```python
from build123d import *

# Parameters (mm, degrees)
SKETCH1_W           = 28.4
SKETCH1_H           = 40.1
BOSS_EXTRUDE1_DEPTH = 4.75
SKETCH2_W           = 3.4
SKETCH2_H           = 23.1
SKETCH2_H_2         = 30.1
CUT_EXTRUDE1_DEPTH  = 26.024088395
SKETCH4_W           = 13.85
SKETCH4_H           = 38.1
SKETCH4_W_2         = 7.85
SKETCH4_H_2         = 30.1
BOSS_EXTRUDE2_DEPTH = 4


with BuildPart() as part:
    # Sketch1 → Boss-Extrude1 (new body)
    with BuildSketch(Plane.XY):
        Rectangle(SKETCH1_W, SKETCH1_H)
    extrude(amount=BOSS_EXTRUDE1_DEPTH)

    # Sketch2 → Cut-Extrude1 (cut, through all)
    with BuildSketch(Plane.XY.offset(4.75)):
        with Locations((10.5, 0)):
            Rectangle(SKETCH2_W, SKETCH2_H)
        with Locations((-10.5, 0)):
            Rectangle(SKETCH2_W, SKETCH2_H)
        Rectangle(SKETCH2_W, SKETCH2_H_2)
    extrude(amount=-CUT_EXTRUDE1_DEPTH, mode=Mode.SUBTRACT)

    # Sketch4 → Boss-Extrude2 (add)
    with BuildSketch(Plane(origin=(0, 0, 0), x_dir=(-1, 0, 0), z_dir=(0, 0, -1))):
        with Locations((0, 1)):
            Rectangle(SKETCH4_W, SKETCH4_H)
        Rectangle(SKETCH4_W_2, SKETCH4_H_2, mode=Mode.SUBTRACT)
    extrude(amount=BOSS_EXTRUDE2_DEPTH)


solid = part.part
```
Can you work these out from the model? Positions are in its coordinate system, mm. A direction names the side the tool comes from. Round coordinates to 2 decimals unless told otherwise and drop trailing zeros. Loops run counter-clockwise (first coordinate to the right, second up) from the corner with the lowest first, then second, coordinate; pieces in that order, holes last. Notation, with made-up numbers: (0, 62.25) -> (37, 62.25) arc R26 cw to (37, 93.25) -> close; hole circle Ø1 at (-28.5, 49). An arc over 180 degrees is marked (long way). One line per item, written item: value. Start each with the question number.
1. If we section it at B-B, the plane y = -8.5: Write out the boundary of the cut face in (x, z) (3 decimals), then the cut area to 3 significant figures.
2. For faces 1 (the flat face through (0, 15.05, -1)), 2 (the flat face through (0, -18.05, -2)), 3 (the flat face through (-11, -11.55, 2)), 4 (the flat face through (6.925, 1, -2)), which set-ups out of +Z, -Z, +X, -X, +Y, -Y let a thin tool reach every point of the face, with its end or its side?
3. If we section it at D-D, the plane z = 2.75: Write out the boundary of the cut face in (x, y), then the cut area to 3 significant figures.
4. If we section it at A-A, the plane y = -14: Write out the boundary of the cut face in (x, z) (3 decimals).
5. If I drill on probe 1 along X at (y, z) = (-4, 4); probe 2 along X at (y, z) = (12.5, 3.5); probe 3 along X at (y, z) = (13, -2) (3 decimals), over which ranges is the centre line in solid material (lowest first)?
6. For pin 1 (2 mm diameter, centred on x = -1, z = -1.5, fed in from -Y); pin 2 (1.5 mm diameter, centred on y = -9, z = -0.5, fed in from +X); pin 3 (3 mm diameter, centred on y = -3, z = -2, fed in from +X) (3 decimals); pin 4 (0.7 mm diameter, centred on x = -3, y = -2.5, fed in from -Z), each with a flat end and sliding along its axis, tell me the tip position at first contact or that it passes through.
7. If we mould it in two halves opening along X, with no side actions, what happens to faces 5 (the flat face through (14.2, 0, 2)), 6 (the flat face through (-7.4, 1.6, 0)), 7 (the flat face through (3, 0, 0)), 8 (the flat face through (-14.2, 0, 2))? For each: pulls with the +X half, pulls with the -X half, needs draft (parallel to the pull), parting line crosses it, or undercut.
8. If we section it at C-C, the plane x = -0.25: Write out the boundary of the cut face in (y, z), then the cut area to 3 significant figures.
Calculated:
1. outline: (-14.2, 0) -> (-12.2, 0) -> (-12.2, 4.75) -> (-14.2, 4.75) -> close; (-8.8, 0) -> (-6.925, 0) -> (-6.925, -4) -> (-3.925, -4) -> (-3.925, 0) -> (-1.7, 0) -> (-1.7, 4.75) -> (-8.8, 4.75) -> close; (1.7, 0) -> (3.925, 0) -> (3.925, -4) -> (6.925, -4) -> (6.925, 0) -> (8.8, 0) -> (8.8, 4.75) -> (1.7, 4.75) -> close; (12.2, 0) -> (14.2, 0) -> (14.2, 4.75) -> (12.2, 4.75) -> close
1. area: 110 mm²
2. face 1: -Z
2. face 2: -Z, +X, -X, -Y
2. face 3: +Z, -Z
2. face 4: -Z, +X, +Y, -Y
3. outline: (-14.2, -20.05) -> (14.2, -20.05) -> (14.2, 20.05) -> (-14.2, 20.05) -> close; hole (-12.2, -11.55) -> (-8.8, -11.55) -> (-8.8, 11.55) -> (-12.2, 11.55) -> close; hole (-1.7, -15.05) -> (1.7, -15.05) -> (1.7, 15.05) -> (-1.7, 15.05) -> close; hole (8.8, -11.55) -> (12.2, -11.55) -> (12.2, 11.55) -> (8.8, 11.55) -> close
3. area: 879 mm²
4. outline: (-14.2, 0) -> (-6.925, 0) -> (-6.925, -4) -> (-3.925, -4) -> (-3.925, 0) -> (-1.7, 0) -> (-1.7, 4.75) -> (-14.2, 4.75) -> close; (1.7, 0) -> (3.925, 0) -> (3.925, -4) -> (6.925, -4) -> (6.925, 0) -> (14.2, 0) -> (14.2, 4.75) -> (1.7, 4.75) -> close
5. probe 1: x = -14.2 to -12.2, -8.8 to -1.7, 1.7 to 8.8, 12.2 to 14.2
5. probe 2: x = -14.2 to -1.7, 1.7 to 14.2
5. probe 3: x = -6.925 to -3.925, 3.925 to 6.925
6. pin 1: stops at y = -18.05
6. pin 2: stops at x = 14.2
6. pin 3: stops at x = 6.925
6. pin 4: stops at z = 0
7. face 5: pulls with the +X half
7. face 6: needs draft
7. face 7: undercut
7. face 8: pulls with the -X half
8. outline: (-20.05, 0) -> (-18.05, 0) -> (-18.05, -4) -> (-15.05, -4) -> (-15.05, 4.75) -> (-20.05, 4.75) -> close; (15.05, -4) -> (20.05, -4) -> (20.05, 4.75) -> (15.05, 4.75) -> close
8. area: 79.5 mm²
